```python
from build123d import *

# Parameters (mm, degrees)
SKETCH1_R               = 1.65
BOSS_EXTRUDE1_DEPTH     = 24
CUT_EXTRUDE1_DEPTH      = 4.5
CUT_EXTRUDE1_DEPTH_BACK = 4.5
CUT_EXTRUDE3_DEPTH      = 10.5
CUT_EXTRUDE3_DEPTH_BACK = 10.5
CUT_EXTRUDE2_DEPTH      = 33.202484376
BOSS_EXTRUDE2_DEPTH     = 1.5
BOSS_EXTRUDE3_START     = 1.5
BOSS_EXTRUDE3_DEPTH     = 1.5
CHAMFER1_SIZE           = 1.5
SKETCH7_R               = 10.5
CUT_EXTRUDE4_DEPTH      = 32.192947921


with BuildPart() as part:
    # Sketch1 → Boss-Extrude1 (new body)
    with BuildSketch(Plane.XY):
        with BuildLine():
            Line((-18.863703305, -1.03527618), (-17.533409567, -6))
            Line((-17.533409567, -6), (18, -6))
            Line((18, -6), (18, 4))
            Line((18, 4), (-15, 4))
            ThreePointArc((-15, 4), (-18.173413361, 2.435045716), (-18.863703305, -1.03527618))
        make_face()
        with Locations((-15, 0)):
            Circle(SKETCH1_R, mode=Mode.SUBTRACT)
    extrude(amount=BOSS_EXTRUDE1_DEPTH)

    # Sketch2 → Cut-Extrude1 (cut, two sides: drawn at the far end of the back side and taken through both)
    with BuildSketch(Plane.XY.offset(12).offset(-CUT_EXTRUDE1_DEPTH_BACK)):
        with BuildLine():
            Line((-11.901189968, -2.421210935), (-19.809111658, -31.933976465))
            Line((-19.809111658, -31.933976465), (-19.809111658, 9.8))
            Line((-19.809111658, 9.8), (9.8, 9.8))
            Line((9.8, 9.8), (9.8, 0))
            ThreePointArc((9.8, 0), (1.220098284, -9.723752371), (-9.496195955, -2.421210935))
            Line((-9.496195955, -2.421210935), (-11.901189968, -2.421210935))
        make_face()
    extrude(amount=CUT_EXTRUDE1_DEPTH + CUT_EXTRUDE1_DEPTH_BACK, mode=Mode.SUBTRACT)

    # Sketch4 → Cut-Extrude3 (cut, two sides: drawn at the far end of the back side and taken through both)
    with BuildSketch(Plane.XY.offset(12).offset(-CUT_EXTRUDE3_DEPTH_BACK)):
        with BuildLine():
            Line((-3.1, 0), (-3.1, 6.453034263))
            Line((-3.1, 6.453034263), (3.1, 6.453034263))
            Line((3.1, 6.453034263), (3.1, 0))
            ThreePointArc((3.1, 0), (0, -3.1), (-3.1, 0))
        make_face()
    extrude(amount=CUT_EXTRUDE3_DEPTH + CUT_EXTRUDE3_DEPTH_BACK, mode=Mode.SUBTRACT)

    # Sketch3 → Cut-Extrude2 (cut, through all)
    with BuildSketch(Plane.XZ.offset(6)):
        with BuildLine():
            Line((13.75, 17.85), (12.25, 17.85))
            ThreePointArc((12.25, 17.85), (10.6, 19.5), (12.25, 21.15))
            Line((12.25, 21.15), (13.75, 21.15))
            ThreePointArc((13.75, 21.15), (15.4, 19.5), (13.75, 17.85))
        make_face()
        with BuildLine():
            Line((13.75, 6.15), (12.25, 6.15))
            ThreePointArc((12.25, 6.15), (10.6, 4.5), (12.25, 2.85))
            Line((12.25, 2.85), (13.75, 2.85))
            ThreePointArc((13.75, 2.85), (15.4, 4.5), (13.75, 6.15))
        make_face()
    extrude(amount=-CUT_EXTRUDE2_DEPTH, mode=Mode.SUBTRACT)

    # Sketch5 → Boss-Extrude2 (add)
    with BuildSketch(Plane.XY.offset(7.5)):
        with BuildLine():
            Line((-3.1, 0), (-3.1, 3.261901286))
            ThreePointArc((-3.1, 3.261901286), (0, -4.5), (3.1, 3.261901286))
            Line((3.1, 3.261901286), (3.1, 0))
            ThreePointArc((3.1, 0), (0, -3.1), (-3.1, 0))
        make_face()
    extrude(amount=BOSS_EXTRUDE2_DEPTH)

    # Sketch6 → Boss-Extrude3 (add)
    with BuildSketch(Plane(origin=(0, 0, 16.5), x_dir=(-1, 0, 0), z_dir=(0, 0, -1)).offset(BOSS_EXTRUDE3_START)):
        with BuildLine():
            Line((-3.1, 0), (-3.1, 3.261901286))
            ThreePointArc((-3.1, 3.261901286), (0, -4.5), (3.1, 3.261901286))
            Line((3.1, 3.261901286), (3.1, 0))
            ThreePointArc((3.1, 0), (0, -3.1), (-3.1, 0))
        make_face()
    extrude(amount=-BOSS_EXTRUDE3_DEPTH)

    # Chamfer1
    chamfer1_edges = [part.edges().sort_by_distance(p)[0] for p in [
        (0, -4.5, 7.5),
        (0, -4.5, 16.5),
    ]]
    chamfer(chamfer1_edges, length=CHAMFER1_SIZE - 0.0001)  # a hair under: the kernel refuses the full size

    # Sketch7 → Cut-Extrude4 (cut, through all)
    with BuildSketch(Plane.XY.offset(24)):
        with Locations((0, 13.27)):
            Circle(SKETCH7_R)
    extrude(amount=-CUT_EXTRUDE4_DEPTH, mode=Mode.SUBTRACT)


solid = part.part
```
Here's how the part is built. I have some questions about the finished solid (model axes, mm). A direction names the side the tool comes from. Give positions to 0.01 mm unless a question says otherwise; leave off trailing zeros. Write each loop counter-clockwise with the first axis right and the second up, starting at its lowest first coordinate (ties: lowest second). Pieces come first, ordered by that corner, then holes. Notation, with made-up numbers: (-25.75, 19.25) -> (21.25, 19.25) arc R17 ccw to (21.25, 44.25) -> close; hole circle Ø4 at (-36, 80.5). An arc over 180 degrees is marked (long way). Use one line per item in the form item = value.
1) We'd pull the mould along X, two halves only. Please class faces 5 (the face through (0, 0, 1.5)), 6 (the face through (-11, -2.421, 12)), 7 (the face through (-18.14, 2.48, 3.7)), 8 (the face through (10.6, -1.1, 4.5)): +X half, -X half, draft (parallel to the pull), parting line (faces both ways), or undercut.
Verdict:
face_5 = undercut
face_6 = draft
face_7 = -X half
face_8 = undercut
2) Suppose I cut it at C-C (y = -5.5). Give the number of separate pieces and of enclosed holes in the cut face, and give its area (3 significant figures).
Verdict:
separate_pieces = 1
enclosed_holes = 3
area = 642 mm2
3) If I drill on L1, parallel to Z at x = 13.5, y = 2; L2, parallel to X at y = 0, z = 21.5; L3, parallel to Y at x = -15, z = 19.25, over which ranges is the centre line in solid material (lowest first)? Write a range as [from, to].
Verdict:
L1 = [0, 2.85], [6.15, 17.85], [21.15, 24]
L2 = [-19, -16.65], [-13.35, -3.1], [3.1, 18]
L3 = [-6, -1.65], [1.65, 4]
4) I'm going to push flat-ended pins straight in: pin 1 (1.6 mm diameter, centred on y = 1, z = 18.5, fed in from -X) (3 decimals); pin 2 (1.2 mm diameter, centred on x = -10.5, z = 11, fed in from +Y). Where does each tip first touch, or does it pass through?
Verdict:
pin_1 = -18.995
pin_2 = -2.42
5) Suppose I cut it at B-B (z = 14.5). Please give me the cut outline in (x, y).
Verdict:
outline = (-12.86, -6) -> (-7.75, -6) arc R9.8 cw to (-9.5, -2.42) -> (-11.9, -2.42) -> close; (7.75, -6) -> (18, -6) -> (18, 4) -> (9.8, 4) -> (9.8, 0) arc R9.8 cw to start
6) On a 3-axis mill with a long thin cutter (end or side, diameter ignored), from which of +Z, -Z, +X, -X, +Y, -Y can I reach the whole of each face in a straight line? I mean faces 1 (the face through (0.16, -4.76, 15.26)), 2 (the face through (10.6, -1.1, 19.5)), 3 (the face through (-12.374, -4.186, 11.937)), 4 (the face through (0, 0, 22.5)). Say none if no direction works.
Verdict:
face_1 = none
face_2 = +Y, -Y
face_3 = -X, +Y
face_4 = +Y
7) Suppose I cut it at A-A (z = 19.5). Please give me the cut outline in (x, y), and give its area (3 significant figures).
Verdict:
outline = (-18.86, -1.04) -> (-17.53, -6) -> (10.6, -6) -> (10.6, 4) -> (4.93, 4) arc R10.5 cw to (3.1, 3.24) -> (3.1, 0) arc R3.1 cw to (-3.1, 0) -> (-3.1, 3.24) arc R10.5 cw to (-4.93, 4) -> (-15, 4) arc R4 ccw to start; (15.4, -6) -> (18, -6) -> (18, 4) -> (15.4, 4) -> close; hole circle Ø3.3 at (-15, 0)
area = 265 mm2
